Here's the drawing with two shaded views (mm, measured from the low corner). I have some questions. A direction names the side the tool comes from. Coordinates: 2 decimals unless noted, no trailing zeros. Order: outer loops, then holes, each group sorted by start corner. A loop starts at its lowest first (then second) coordinate and runs counter-clockwise, first axis right, second up. Notation, with made-up numbers: (71.5, 78.5) -> (101.5, 78.5) arc R16 cw to (101.5, 107.5) -> close; hole circle Ø7 at (77, 73). An arc over 180 degrees is marked (long way). Answer as a JSON object with one key per item and string values. Group by question number.
(1) Which directions (+Z, -Z, +X, -X, +Y, -Y) give clear straight access to the entire face, cutting with the end or side of a thin tool? Please do the marked faces 4 and 5.
(2) If we mould it in two halves opening along Y, with no side actions, what happens to the marked faces 1, 2 and 3? For each: pulls with the +Y half, pulls with the -Y half, needs draft (parallel to the pull), parting line crosses it, or undercut.
(3) I need wall thicknesses on line 1 (Y direction, x = 21.5, z = 21.5); line 2 (X direction, y = 4.5, z = 18). Which ranges of each line are inside material? Lowest first, please.
(4) I want a section at A-A, the plane z = 14. List the corners of the cut face in (x, y) for me.
(5) I want a section at C-C, the plane x = 33.5. List the corners of the cut face in (y, z) for me.
(6) I want a section at B-B, the plane y = 30. List the corners of the cut face in (x, z) for me, plus the area to 3 significant figures.
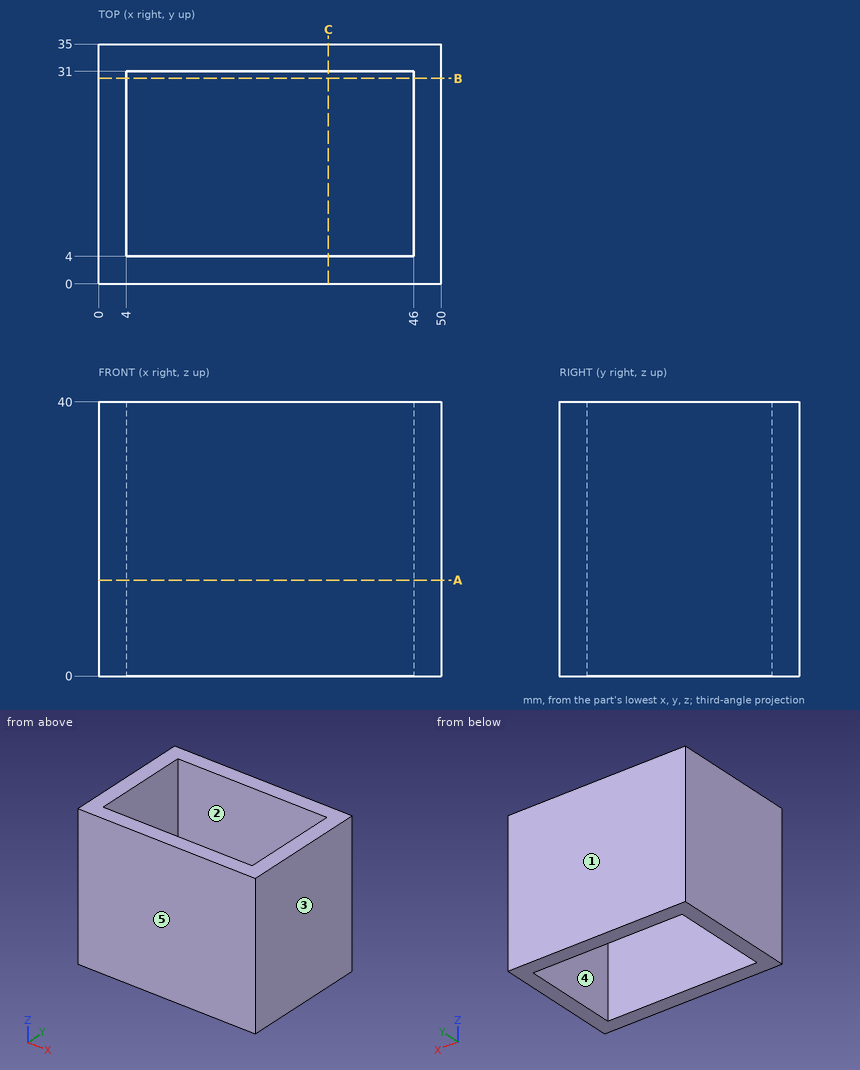
Computed values:
{
 "1": {"face 4": "+Z, -Z", "face 5": "+Z, -Z, +X, -X, -Y"},
 "2": {"face 1": "pulls with the +Y half", "face 2": "undercut", "face 3": "needs draft"},
 "3": {"line 1": "y = 0 to 4, 31 to 35", "line 2": "x = 0 to 4, 46 to 50"},
 "4": {"outline": "(0, 0) -> (50, 0) -> (50, 35) -> (0, 35) -> close; hole (4, 4) -> (46, 4) -> (46, 31) -> (4, 31) -> close"},
 "5": {"outline": "(0, 0) -> (4, 0) -> (4, 40) -> (0, 40) -> close; (31, 0) -> (35, 0) -> (35, 40) -> (31, 40) -> close"},
 "6": {"outline": "(0, 0) -> (4, 0) -> (4, 40) -> (0, 40) -> close; (46, 0) -> (50, 0) -> (50, 40) -> (46, 40) -> close", "area": "320 mm2"}
}
